Here's how the part is built. I have some questions about the finished solid (model axes, mm). Face numbers are marked on the shaded views. Coordinates: 2 decimals unless noted, no trailing zeros. Write each loop counter-clockwise with the first axis right and the second up, starting at its lowest first coordinate (ties: lowest second). Pieces come first, ordered by that corner, then holes.
Item 1: We'd pull the mould along Z, two halves only. Please class the marked faces 1, 2 and 3: +Z half, -Z half, draft (parallel to the pull), parting line (faces both ways), or undercut.
Item 2: If I drill on line 1 (Y direction, x = 6.5, z = 0) (1 decimal); line 2 (Y direction, x = 95, z = 0.5); line 3 (Y direction, x = 6.5, z = 1.25), over which ranges is the centre line in solid material (lowest first)?
Item 3: If we section it at B-B (x = 35.5): Please give me the cut outline in (y, z).
Item 4: If we section it at A-A (y = 0): Please give me the cut outline in (x, z) (3 decimals).
Item 5: I'm going to push flat-ended pins straight in: pin 1 Ø0.8 at (x, z) = (94.5, 2) entering from +Y; pin 2 Ø5 at (y, z) = (0, -0.5) entering from -X (3 decimals). Where does each tip first touch, or does it pass through?
from build123d import *

# Parameters (mm, degrees)
SKETCH1_W           = 12.6492
SKETCH1_H           = 15.875
BOSS_EXTRUDE1_DEPTH = 111.125
HOLE1_D             = 6.35
HOLE1_DEPTH         = 15.875
CUT_EXTRUDE1_START  = -13.6492
CUT_EXTRUDE1_DEPTH  = 14.6492
LPATTERN2_COUNT     = 13
LPATTERN2_PITCH     = 6.6548
CHAMFER1_SIZE       = 1.524


with BuildPart() as part:
    # Sketch1 → Boss-Extrude1 (new body)
    with BuildSketch(Plane(origin=(0, 0, 0), x_dir=(0, 0, -1), z_dir=(1, 0, 0))):
        Rectangle(SKETCH1_W, SKETCH1_H)
    extrude(amount=BOSS_EXTRUDE1_DEPTH)

    # Hole1
    with Locations(Plane.ZY):
        with Locations((0, 0)):
            Hole(HOLE1_D / 2, depth=HOLE1_DEPTH)

    # Sketch4 → Cut-Extrude1 (cut)
    with BuildSketch(Plane.XY.offset(6.3246).offset(CUT_EXTRUDE1_START)):
        Polygon((-48.282488077, 192.931990587), (19.05, 7.9375), (20.704827067, 3.3909), (23.244827067, 3.3909), (24.899654134, 7.9375), (92.232142211, 192.931990587), (92.232142211, 586.666040414), (-48.282488077, 586.666040414), align=None)
    cut_extrude1 = extrude(amount=CUT_EXTRUDE1_DEPTH, mode=Mode.SUBTRACT)

    # LPattern2: Cut-Extrude1 ×13
    with Locations(*[(i * LPATTERN2_PITCH, 0, 0) for i in range(1, LPATTERN2_COUNT)]):
        add(cut_extrude1, mode=Mode.SUBTRACT)

    # Chamfer1
    chamfer1_edges = [part.edges().sort_by_distance(p)[0] for p in [
        (111.125, 0, 6.3246),
        (111.125, -7.9375, 0),
        (111.125, 0, -6.3246),
        (111.125, 7.9375, 0),
    ]]
    chamfer(chamfer1_edges, length=CHAMFER1_SIZE)


solid = part.part
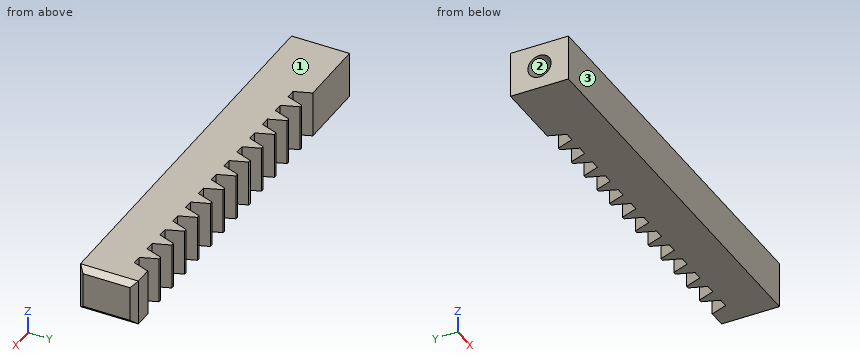
Answer list:
1. face 1: +Z half
1. face 2: undercut
1. face 3: draft
2. line 1: y = -7.9 to -3.2, 3.2 to 7.9
2. line 2: y = -7.94 to 3.39
2. line 3: y = -7.94 to -2.92, 2.92 to 7.94
3. outline: (-7.94, -6.32) - (3.39, -6.32) - (3.39, 6.32) - (-7.94, 6.32) - close
4. outline: (0, -6.325) - (109.601, -6.325) - (111.125, -4.801) - (111.125, 4.801) - (109.601, 6.325) - (0, 6.325) - (0, 3.175) - (15.875, 3.175) - (15.875, -3.175) - (0, -3.175) - close
5. pin 1: stops at y = 3.39
5. pin 2: stops at x = 15.875
